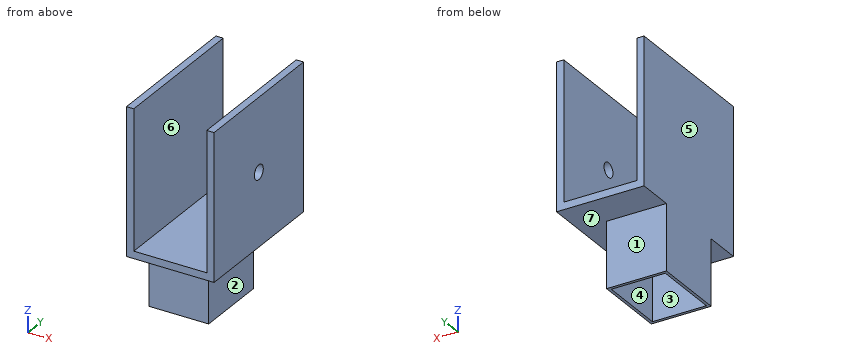
```python
from build123d import *

# Parameters (mm, degrees)
SCHIZZO1_W                   = 60
SCHIZZO1_H                   = 100
ESTRUSIONE_ESTRUSIONE1_DEPTH = 100
SCHIZZO2_W                   = 50
SCHIZZO2_H                   = 95
TAGLIO_ESTRUSIONE1_DEPTH     = 101
SCHIZZO3_R                   = 5
TAGLIO_ESTRUSIONE2_DEPTH     = 21
SCHIZZO4_W                   = 41
SCHIZZO4_H                   = 50
ESTRUSIONE_ESTRUSIONE2_DEPTH = 45
SVUOTA1_T                    = -2


with BuildPart() as part:
    # Schizzo1 → Estrusione-Estrusione1 (new body)
    with BuildSketch(Plane.XY):
        Rectangle(SCHIZZO1_W, SCHIZZO1_H)
    extrude(amount=ESTRUSIONE_ESTRUSIONE1_DEPTH)

    # Schizzo2 → Taglio-Estrusione1 (cut, through all)
    with BuildSketch(Plane(origin=(0, 50, 0), x_dir=(1, 0, 0), z_dir=(0, 1, 0))):
        with Locations((0, -52.5)):
            Rectangle(SCHIZZO2_W, SCHIZZO2_H)
    extrude(amount=-TAGLIO_ESTRUSIONE1_DEPTH, mode=Mode.SUBTRACT)

    # Schizzo3 → Taglio-Estrusione2 (cut)
    with BuildSketch(Plane(origin=(30, 0, 0), x_dir=(0, 0, -1), z_dir=(1, 0, 0))):
        with Locations((-50, 0)):
            Circle(SCHIZZO3_R)
    extrude(amount=-TAGLIO_ESTRUSIONE2_DEPTH, mode=Mode.SUBTRACT)

    # Schizzo4 → Estrusione-Estrusione2 (add)
    with BuildSketch(Plane(origin=(0, 0, 0), x_dir=(-1, 0, 0), z_dir=(0, 0, -1))):
        with Locations((9.5, 0)):
            Rectangle(SCHIZZO4_W, SCHIZZO4_H)
    extrude(amount=ESTRUSIONE_ESTRUSIONE2_DEPTH)

    # Svuota1
    svuota1_openings = [part.faces().sort_by_distance(p)[0] for p in [
        (-9.5, 0, -45),
    ]]
    offset(amount=SVUOTA1_T, openings=svuota1_openings, kind=Kind.INTERSECTION)


solid = part.part
```
For this review, take the finished solid that the model builds, in its own axes (mm). Face numbers are marked on the shaded views. A direction names the side the tool comes from. Round coordinates to 2 decimals unless told otherwise and drop trailing zeros. Write each loop counter-clockwise with the first axis right and the second up, starting at its lowest first coordinate (ties: lowest second). Pieces come first, ordered by that corner, then holes. Notation, with made-up numbers: (34.25, 88.5) - (91.25, 88.5) arc R10 cw to (91.25, 93.5) - close; hole circle Ø4 at (80.25, -9). An arc over 180 degrees is marked (long way). Answer as a JSON object with one key per item and string values.
1. To check wall thickness, follow line 1 along X through (y, z) = (37, 46); line 2 along Y through (x, z) = (2, -37.5); line 3 along Y through (x, z) = (26.4, 50). State the ranges of each line that lie inside material, in increasing order.
Response values:
{"line 1": "x = -30 to -28, -27 to -25, 25 to 27, 28 to 30", "line 2": "y = -25 to -23, 23 to 25", "line 3": "y = -50 to -5, 5 to 50"}
2. Draft analysis for pull direction X (two halves, no side actions). For the marked faces 4, 5, 6 and 7, state which applies: +X half, -X half, draft (parallel to the pull), parting line (faces both ways), or undercut.
Response values:
{"face 4": "undercut", "face 5": "-X half", "face 6": "undercut", "face 7": "draft"}
3. Tool access review of the marked faces 1, 2 and 3: name each direction out of +Z, -Z, +X, -X, +Y, -Y from which nothing blocks a thin tool from reaching the whole face with its end or side.
Response values:
{"face 1": "-Z, +X, -X, +Y", "face 2": "-Z, +X, +Y, -Y", "face 3": "-Z"}
4. We need section C-C on y = 31. Give the boundary of the cut face in (x, z).
Response values:
{"outline": "(-30, 0) - (30, 0) - (30, 100) - (25, 100) - (25, 5) - (-25, 5) - (-25, 100) - (-30, 100) - close; hole (-28, 2) - (28, 2) - (28, 98) - (27, 98) - (27, 3) - (-27, 3) - (-27, 98) - (-28, 98) - close"}
5. We need section B-B on y = 0. Give the boundary of the cut face in (x, z), then the cut area to 3 significant figures.
Response values:
{"outline": "(-30, -45) - (-28, -45) - (-28, 98) - (-27, 98) - (-27, 3) - (27, 3) - (27, 43) - (28, 43) - (28, 2) - (9, 2) - (9, -45) - (11, -45) - (11, 0) - (30, 0) - (30, 45) - (25, 45) - (25, 5) - (-25, 5) - (-25, 100) - (-30, 100) - close; (25, 55) - (30, 55) - (30, 100) - (25, 100) - close; hole (27, 57) - (28, 57) - (28, 98) - (27, 98) - close", "area": "1,070 mm2"}
6. We need section A-A on z = 50. Give the boundary of the cut face in (x, y), then the cut area to 3 significant figures.
Response values:
{"outline": "(-30, -50) - (-25, -50) - (-25, 50) - (-30, 50) - close; (25, -50) - (30, -50) - (30, -5) - (25, -5) - close; (25, 5) - (30, 5) - (30, 50) - (25, 50) - close; hole (-28, -48) - (-27, -48) - (-27, 48) - (-28, 48) - close; hole (27, -48) - (28, -48) - (28, -7) - (27, -7) - close; hole (27, 7) - (28, 7) - (28, 48) - (27, 48) - close", "area": "772 mm2"}
7. For pin 1 Ø12.5 at (x, z) = (-17.5, -33) entering from -Y; pin 2 Ø18.5 at (x, z) = (-13.5, -15) entering from +Y; pin 3 Ø5 at (x, y) = (15, 30.5) entering from -Z, all flat-tipped, find the tip position at first contact; note any pin that passes through.
Response values:
{"pin 1": "stops at y = -25", "pin 2": "stops at y = 25", "pin 3": "stops at z = 0"}
8. We need section D-D on x = 5. Give the boundary of the cut face in (y, z).
Response values:
{"outline": "(-50, 0) - (-25, 0) - (-25, -45) - (-23, -45) - (-23, 2) - (-48, 2) - (-48, 3) - (48, 3) - (48, 2) - (23, 2) - (23, -45) - (25, -45) - (25, 0) - (50, 0) - (50, 5) - (-50, 5) - close"}
